Source: three-view drawing plus pictorial views. Frame: mm from the lowest corner of the part. A direction names the side the tool comes from. Give positions to 0.01 mm unless a question says otherwise; leave off trailing zeros. Order: outer loops, then holes, each group sorted by start corner. A loop starts at its lowest first (then second) coordinate and runs counter-clockwise, first axis right, second up. Notation, with made-up numbers: M 71.5,19.25 L 124.5,19.25 A17 ccw 124.5,38.25 Z; hole C 17.5,17 d8. An arc over 180 degrees is marked long. Use CSV: the item, a comma, the result in double quotes.
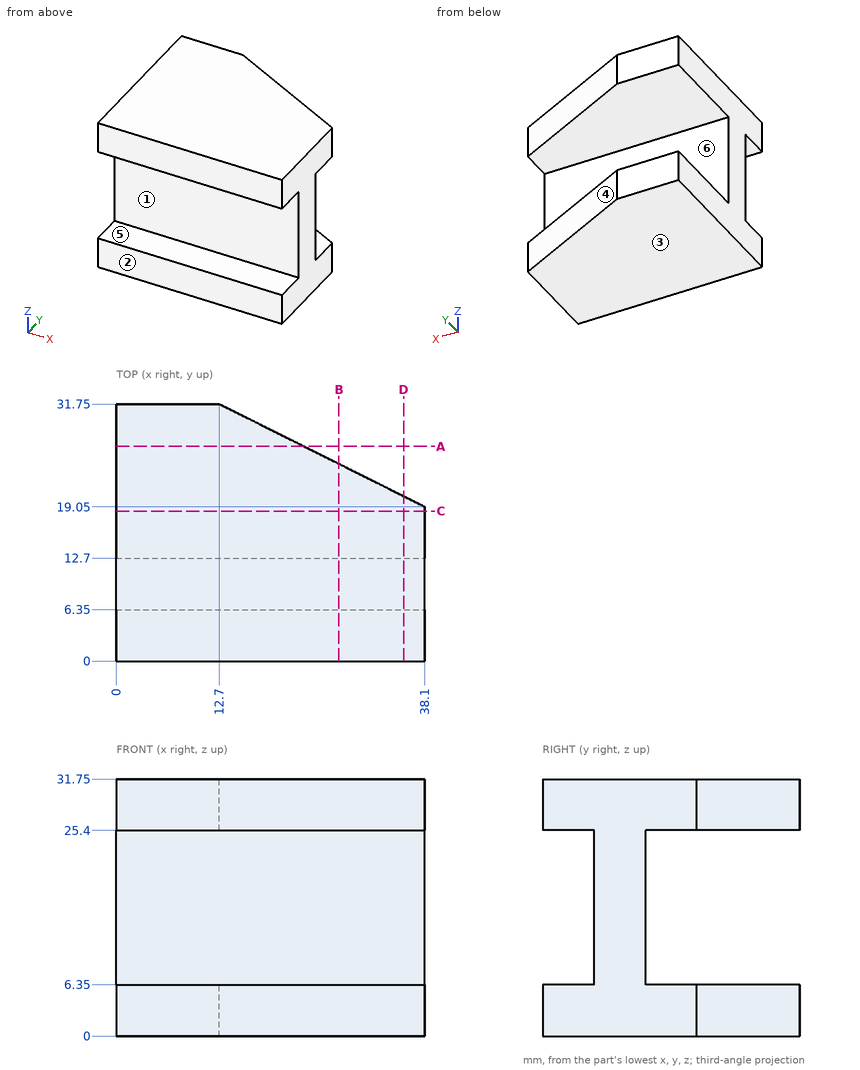
1. Section C-C, the plane y = 18.5. Return the cut outline in (x, z), plus the area to 3 significant figures.
Answer:
outline,"M 0,0 L 38.1,0 L 38.1,6.35 L 0,6.35 Z; M 0,25.4 L 38.1,25.4 L 38.1,31.75 L 0,31.75 Z"
area,"484 mm2"
2. Pull-direction query (Z, two-part tool) for the marked faces 1, 2 and 3; classes: +Z half, -Z half, draft (parallel to the pull), parting line (faces both ways), or undercut.
Answer:
face 1,"undercut"
face 2,"draft"
face 3,"-Z half"
3. Line query: line 1 (Z direction, x = 26.5, y = 16); line 2 (Y direction, x = 3, z = 19). Output: solid intervals per line, ascending.
Answer:
line 1,"0 to 6.35, 25.4 to 31.75"
line 2,"6.35 to 12.7"
4. Reachability of the marked faces 4, 5 and 6 from +Z, -Z, +X, -X, +Y, -Y: full face, straight path, thin tool, end or side. Return the list, or none.
Answer:
face 4,"+Z, -Z, +X, +Y"
face 5,"+X, -X, -Y"
face 6,"+X, -X, +Y"
5. Section D-D, the plane x = 35.5. Return the cut outline in (y, z), plus the area to 3 significant figures.
Answer:
outline,"M 0,0 L 20.35,0 L 20.35,6.35 L 12.7,6.35 L 12.7,25.4 L 20.35,25.4 L 20.35,31.75 L 0,31.75 L 0,25.4 L 6.35,25.4 L 6.35,6.35 L 0,6.35 Z"
area,"379 mm2"
6. Section B-B, the plane x = 27.5. Return the cut outline in (y, z), plus the area to 3 significant figures.
Answer:
outline,"M 0,0 L 24.35,0 L 24.35,6.35 L 12.7,6.35 L 12.7,25.4 L 24.35,25.4 L 24.35,31.75 L 0,31.75 L 0,25.4 L 6.35,25.4 L 6.35,6.35 L 0,6.35 Z"
area,"430 mm2"
7. Section A-A, the plane y = 26.5. Return the cut outline in (x, z).
Answer:
outline,"M 0,0 L 23.2,0 L 23.2,6.35 L 0,6.35 Z; M 0,25.4 L 23.2,25.4 L 23.2,31.75 L 0,31.75 Z"
8. Pin query (flat end, axial travel): pin 1 Ø9.5 at (x, z) = (11.5, 14) entering from +Y; pin 2 Ø1.5 at (x, z) = (24, 25.5) entering from +Y (3 decimals); pin 3 Ø5.5 at (x, z) = (27.5, 12.5) entering from -Y. Return the tip coordinate at first contact, or that it passes through.
Answer:
pin 1,"y = 12.7"
pin 2,"y = 26.475"
pin 3,"y = 6.35"
